Study the drawing (mm; zero at the part's minimum x, y, z) and answer. A direction names the side the tool comes from. Coordinates: 2 decimals unless noted, no trailing zeros. Loops run counter-clockwise (first coordinate to the right, second up) from the corner with the lowest first, then second, coordinate; pieces in that order, holes last. Notation, with made-up numbers: (86.5, -27) - (116.5, -27) arc R20 cw to (116.5, -11) - close; hole circle Ø1 at (-3.5, 0.25). An arc over 180 degrees is marked (long way). Use CSV: the item, a comma, the result in double quotes.
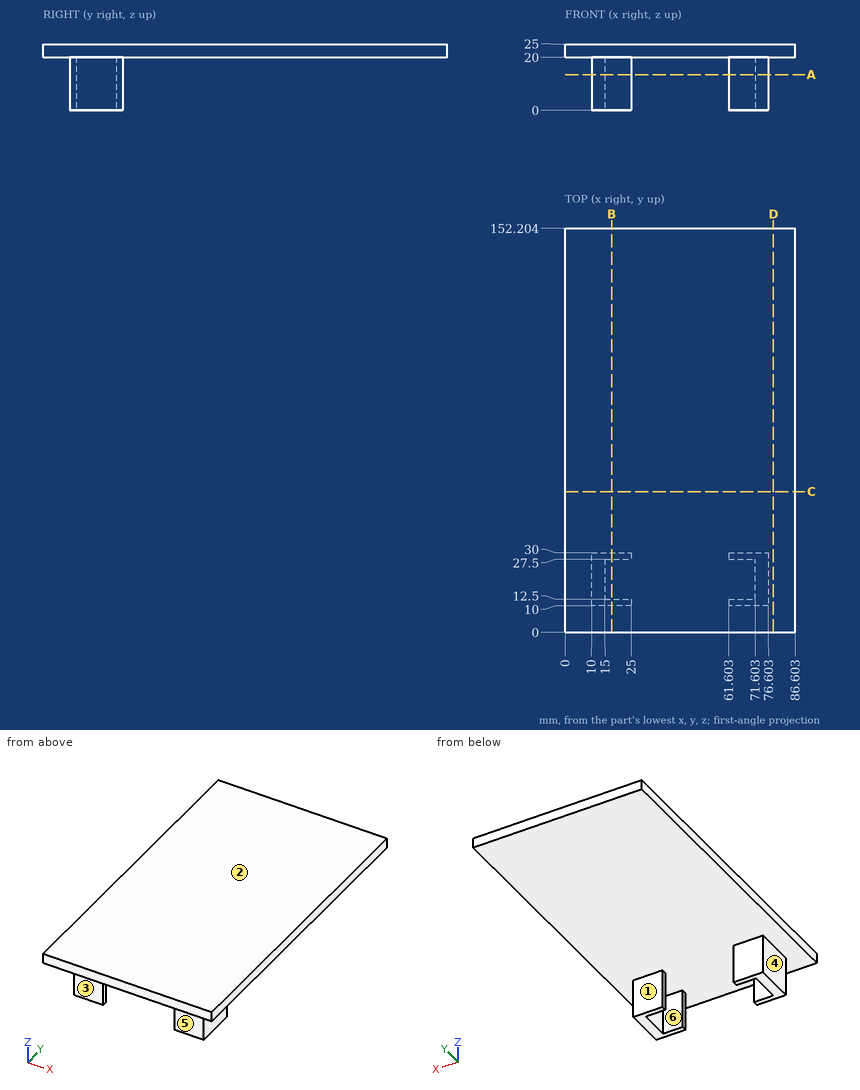
Q1. The part is cut by section C-C on y = 53. Determine the outline of the cut face in (x, z), and give its area (3 significant figures).
Reported:
outline,"(0, 20) - (86.6, 20) - (86.6, 25) - (0, 25) - close"
area,"433 mm²"
Q2. A tool of negligible diameter and unlimited length cuts with its end or side. For the marked faces 1, 2 and 3, from which of +Z, -Z, +X, -X, +Y, -Y can it reach the whole face along a straight path? Write none if from no direction.
Reported:
face 1,"-Z, +X, -X, +Y"
face 2,"+Z, +X, -X, +Y, -Y"
face 3,"-Z, +X, -X, -Y"
Q3. The part is cut by section A-A on z = 13.5. Determine the outline of the cut face in (x, y), and give its area (3 significant figures).
Reported:
outline,"(10, 10) - (25, 10) - (25, 12.5) - (15, 12.5) - (15, 27.5) - (25, 27.5) - (25, 30) - (10, 30) - close; (61.6, 10) - (76.6, 10) - (76.6, 30) - (61.6, 30) - (61.6, 27.5) - (71.6, 27.5) - (71.6, 12.5) - (61.6, 12.5) - close"
area,"300 mm²"
Q4. The part is cut by section B-B on x = 17.5. Determine the outline of the cut face in (y, z), and give its area (3 significant figures).
Reported:
outline,"(0, 20) - (10, 20) - (10, 0) - (12.5, 0) - (12.5, 20) - (27.5, 20) - (27.5, 0) - (30, 0) - (30, 20) - (152.2, 20) - (152.2, 25) - (0, 25) - close"
area,"861 mm²"
Q5. For a pull along Y with two mould halves and no side action, classify the marked faces 4, 5 and 6 as +Y half, -Y half, draft (parallel to the pull), parting line (faces both ways), or undercut.
Reported:
face 4,"draft"
face 5,"-Y half"
face 6,"undercut"
Q6. Given P1, Ø5, axis at x = 17.5, z = 7, coming from the -Y side; P2, Ø1.2, axis at y = 11.5, z = 15, coming from the -X side; P3, Ø2, axis at y = 29.5, z = 6.5, coming from the +X side, each flat-ended and moving along its own axis, determine where each tip first touches the part or whether it passes through.
Reported:
P1,"stops at y = 10"
P2,"stops at x = 10"
P3,"stops at x = 76.6"
Q7. The part is cut by section D-D on x = 78.5. Determine the outline of the cut face in (y, z), and give its area (3 significant figures).
Reported:
outline,"(0, 20) - (152.2, 20) - (152.2, 25) - (0, 25) - close"
area,"761 mm²"
Q8. Find the intervals of material crossed by probe 1 along X at (y, z) = (27, 6.25); probe 2 along Y at (x, z) = (62.5, 11.75); probe 3 along Z at (x, y) = (66, 89), in increasing order. Write a range as [from, to].
Reported:
probe 1,"x = [10, 15], [71.6, 76.6]"
probe 2,"y = [10, 12.5], [27.5, 30]"
probe 3,"z = [20, 25]"
